CAD build for the part. Positions are in the model's coordinates, mm. Face numbers are marked on the shaded views. Give positions to 0.01 mm unless a question says otherwise; leave off trailing zeros. Order: outer loops, then holes, each group sorted by start corner. A loop starts at its lowest first (then second) coordinate and runs counter-clockwise, first axis right, second up. Notation, with made-up numbers: (14.5, 88.25) -> (38.5, 88.25) arc R20 cw to (38.5, 119.25) -> close; hole circle Ø11 at (74.25, 20.25). An arc over 180 degrees is marked (long way). Answer as CSV lines item,"result".
```python
from build123d import *

# Parameters (mm, degrees)
SKETCH1_R               = 12.5
BOSS_EXTRUDE1_DEPTH     = 18
CUT_EXTRUDE1_DEPTH      = 26.228951623
CUT_EXTRUDE1_DEPTH_BACK = 26.228951623
SKETCH2_R               = 10.05
CUT_EXTRUDE2_DEPTH      = 34.24530042
CUT_EXTRUDE2_DEPTH_BACK = 34.24530042
SKETCH6_R               = 1.65


with BuildPart() as part:
    # Sketch1 → Boss-Extrude1 (new body)
    with BuildSketch(Plane.XY):
        Circle(SKETCH1_R)
    extrude(amount=BOSS_EXTRUDE1_DEPTH)

    # Sketch2 → Cut-Extrude1 (cut, two sides: drawn at the far end of the back side and taken through both)
    with BuildSketch(Plane.XY.offset(18).offset(-CUT_EXTRUDE1_DEPTH_BACK)):
        Circle(SKETCH2_R)
    extrude(amount=CUT_EXTRUDE1_DEPTH + CUT_EXTRUDE1_DEPTH_BACK, mode=Mode.SUBTRACT)

    # Sketch6 → Cut-Extrude2 (cut, two sides: drawn at the far end of the back side and taken through both)
    with BuildSketch(Plane(origin=(0, -12.5, 0), x_dir=(-1, 0, 0), z_dir=(0, -1, 0)).offset(-CUT_EXTRUDE2_DEPTH_BACK)):
        with Locations(Location((0, -5, 0), (0, 0, 90))):
            Circle(SKETCH6_R)
    extrude(amount=CUT_EXTRUDE2_DEPTH + CUT_EXTRUDE2_DEPTH_BACK, mode=Mode.SUBTRACT)


solid = part.part
```
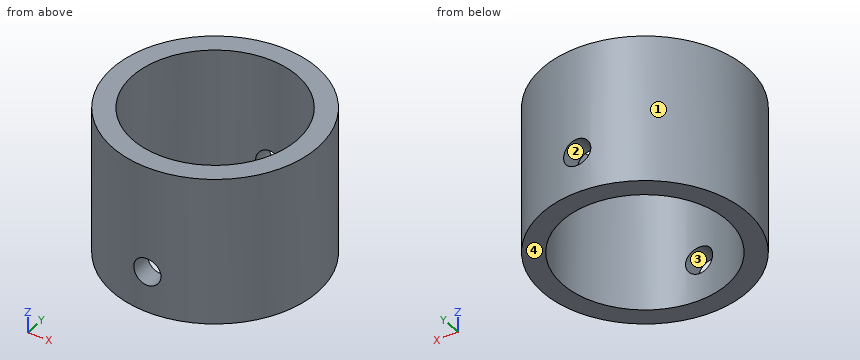
1) Band-saw the part on B-B, the plane x = 0. Write the cut outline in (y, z), then the cut area to 3 significant figures.
Data:
outline,"(-12.5, 0) -> (-10.05, 0) -> (-10.05, 3.35) -> (-12.5, 3.35) -> close; (-12.5, 6.65) -> (-10.05, 6.65) -> (-10.05, 18) -> (-12.5, 18) -> close; (10.05, 0) -> (12.5, 0) -> (12.5, 3.35) -> (10.05, 3.35) -> close; (10.05, 6.65) -> (12.5, 6.65) -> (12.5, 18) -> (10.05, 18) -> close"
area,"72.0 mm2"
2) Band-saw the part on A-A, the plane y = 0. Write the cut outline in (x, z), then the cut area to 3 significant figures.
Data:
outline,"(-12.5, 0) -> (-10.05, 0) -> (-10.05, 18) -> (-12.5, 18) -> close; (10.05, 0) -> (12.5, 0) -> (12.5, 18) -> (10.05, 18) -> close"
area,"88.2 mm2"
3) Pin check, flat tips, straight feed: P1, Ø2, axis at x = 0, z = 5, coming from the +Y side; P2, Ø8, axis at x = -6, z = 2, coming from the +Y side; P3, Ø5, axis at y = 6, z = 10.5, coming from the -X side; P4, Ø2, axis at y = 8.5, z = 13.5, coming from the -X side. Stop position of each tip, or through.
Data:
P1,"passes through"
P2,"stops at y = 12.34"
P3,"stops at x = -12"
P4,"stops at x = -10"
4) Wall check: line 1 along Z through (x, y) = (0, -10.6); line 2 along X through (y, z) = (-0.25, 11.75); line 3 along X through (y, z) = (11, 5). Give the ranges that are in metal, low to high. Write a range as [from, to].
Data:
line 1,"z = [0, 3.35], [6.65, 18]"
line 2,"x = [-12.5, -10.05], [10.05, 12.5]"
line 3,"x = [-5.94, -1.65], [1.65, 5.94]"
5) Band-saw the part on C-C, the plane z = 3.75. Write the cut outline in (x, y).
Data:
outline,"(-1.08, -12.45) -> (-1.08, -9.99) arc R10.05 cw to (-1.08, 9.99) -> (-1.08, 12.45) arc R12.5 ccw to start; (1.08, -12.45) arc R12.5 ccw to (1.08, 12.45) -> (1.08, 9.99) arc R10.05 cw to (1.08, -9.99) -> close"
6) Band-saw the part on D-D, the plane z = 11.75. Write the cut outline in (x, y), then the cut area to 3 significant figures.
Data:
outline,"circle Ø25 at (0, 0); hole circle Ø20.1 at (0, 0)"
area,"174 mm2"
7) Pull direction X, two halves, no side cores. Call the marked faces 1, 2, 3 and 4: pulls with the +X half, pulls with the -X half, needs draft (parallel to the pull), parting line crosses it, or undercut.
Data:
face 1,"parting line crosses it"
face 2,"undercut"
face 3,"undercut"
face 4,"needs draft"
